Source: CAD feature listing. Evaluate the final solid. Frame: model axes, mm. Round coordinates to 2 decimals unless told otherwise and drop trailing zeros. Write each loop counter-clockwise with the first axis right and the second up, starting at its lowest first coordinate (ties: lowest second). Pieces come first, ordered by that corner, then holes. Notation, with made-up numbers: (59, -7) -> (104, -7) arc R17 cw to (104, 0) -> close; hole circle Ø4 at (0.5, -36.5). An arc over 180 degrees is marked (long way). Put each result on its own line as item: value.
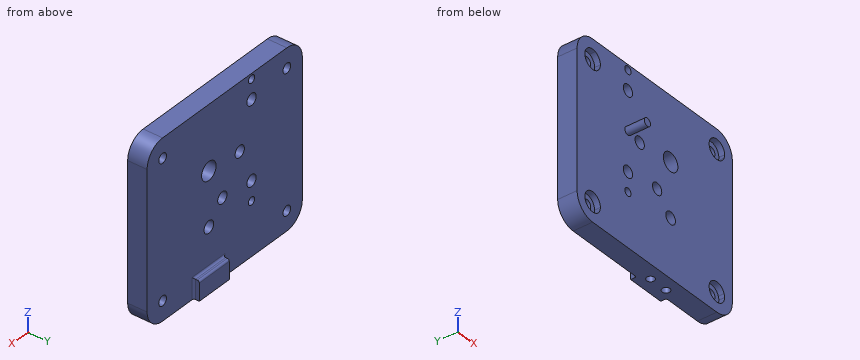
```python
from build123d import *

# Parameters (mm, degrees)
BOSS_EXTRUDE1_DEPTH = 12.7
SKETCH5_R           = 11.9126
SKETCH5_R_2         = 7.9375
SKETCH5_R_3         = 5.9563
CUT_EXTRUDE3_DEPTH  = 231.35713577
CUT_EXTRUDE4_DEPTH  = 231.35713577
CUT_EXTRUDE5_DEPTH  = 7.5057
SKETCH8_R           = 6.35
CUT_EXTRUDE6_DEPTH  = 187.663093698
BOSS_EXTRUDE2_DEPTH = 25.4
SKETCH10_W          = 49.05855317
SKETCH10_H          = 25.4
BOSS_EXTRUDE3_DEPTH = 7.493
FILLET1_R           = 2.54
SKETCH11_R          = 5.08
CUT_EXTRUDE7_DEPTH  = 17.78
SKETCH12_R          = 7.62
CUT_EXTRUDE8_DEPTH  = 188.531502891
SKETCH14_R          = 5.08
BOSS_EXTRUDE4_DEPTH = 50.8
SKETCH16_R          = 7.62
CUT_EXTRUDE10_DEPTH = 193.622803885
SKETCH17_R          = 5.08
CUT_EXTRUDE11_DEPTH = 193.622803885


with BuildPart() as part:
    # Sketch2 → Boss-Extrude1 (new, symmetric)
    with BuildSketch(Plane(origin=(0, 0, 0), x_dir=(1, 0, 0), z_dir=(0, 1, 0))):
        Polygon((114.3, 127), (190.5, 76.2), (190.5, -76.2), (114.3, -127), (-114.3, -127), (-190.5, -76.2), (-190.5, 76.2), (-114.3, 127), align=None)
    extrude(amount=BOSS_EXTRUDE1_DEPTH, both=True)

    # Sketch5 → Cut-Extrude3 (cut, through all)
    # profile 1 of 3: a face of its own
    with BuildSketch(Plane(origin=(0, 12.7, 0), x_dir=(1, 0, 0), z_dir=(0, 1, 0))):
        with Locations(Location((11.947126713, -37.290041101, 0), (0, 0, 270))):
            Circle(SKETCH5_R)
    # profile 2 of 3: a face of its own
    with BuildSketch(Plane(origin=(0, 12.7, 0), x_dir=(1, 0, 0), z_dir=(0, 1, 0))):
        with Locations(Location((11.947126713, 32.712358899, 0), (0, 0, 270))):
            Circle(SKETCH5_R_2)
        with Locations((11.947126713, 32.712358899)):
            Circle(SKETCH5_R_3, mode=Mode.SUBTRACT)
    # profile 3 of 3: a face of its own
    with BuildSketch(Plane(origin=(0, 12.7, 0), x_dir=(1, 0, 0), z_dir=(0, 1, 0))):
        with Locations((11.947126713, 32.712358899)):
            Circle(SKETCH5_R_3)
    extrude(amount=-CUT_EXTRUDE3_DEPTH, mode=Mode.SUBTRACT)

    # Sketch6 → Cut-Extrude4 (cut, through all)
    with BuildSketch(Plane(origin=(0, 12.7, 0), x_dir=(1, 0, 0), z_dir=(0, 1, 0))):
        Polygon((-114.3, -127), (114.3, -127), (190.5, -76.2), (190.5, 76.2), (114.3, 127), (-114.3, 127), (-190.5, 76.2), (-190.5, -76.2), align=None)
        Polygon((-141.354573287, 83.118658899), (-115.954573287, 108.518658899), (87.753426713, 108.518658899), (113.153426713, 83.118658899), (113.153426713, -95.189341101), (87.753426713, -120.589341101), (-115.954573287, -120.589341101), (-141.354573287, -95.189341101), align=None, mode=Mode.SUBTRACT)
    extrude(amount=-CUT_EXTRUDE4_DEPTH, mode=Mode.SUBTRACT)

    # Sketch7 → Cut-Extrude5 (cut)
    with BuildSketch(Plane.XZ.offset(12.7)):
        with BuildLine():
            ThreePointArc((83.29952358, 107.082731992), (78.773170592, 86.20908498), (99.646817604, 90.735437968))
            Line((99.646817604, 90.735437968), (83.29952358, 107.082731992))
        make_face()
        with BuildLine():
            Line((83.29952358, 107.082731992), (99.646817604, 90.735437968))
            ThreePointArc((99.646817604, 90.735437968), (100.250147569, 92.926164607), (100.453426713, 95.189341101))
            ThreePointArc((100.453426713, 95.189341101), (94.989635327, 105.626164607), (83.29952358, 107.082731992))
        make_face()
        with BuildLine():
            ThreePointArc((-103.254573287, 95.189341101), (-105.517749781, 102.425549715), (-111.500670154, 107.082731992))
            Line((-111.500670154, 107.082731992), (-127.847964178, 90.735437968))
            ThreePointArc((-127.847964178, 90.735437968), (-113.691396793, 82.692620245), (-103.254573287, 95.189341101))
        make_face()
        with BuildLine():
            Line((-127.847964178, 90.735437968), (-111.500670154, 107.082731992))
            ThreePointArc((-111.500670154, 107.082731992), (-124.934829408, 104.169597223), (-127.847964178, 90.735437968))
        make_face()
        with BuildLine():
            ThreePointArc((100.453426713, -83.118658899), (100.250147569, -80.855482405), (99.646817604, -78.664755766))
            Line((99.646817604, -78.664755766), (83.29952358, -95.012049789))
            ThreePointArc((83.29952358, -95.012049789), (94.989635327, -93.555482405), (100.453426713, -83.118658899))
        make_face()
        with BuildLine():
            Line((83.29952358, -95.012049789), (99.646817604, -78.664755766))
            ThreePointArc((99.646817604, -78.664755766), (78.773170592, -74.138402777), (83.29952358, -95.012049789))
        make_face()
        with BuildLine():
            ThreePointArc((-127.847964178, -78.664755766), (-124.934829408, -92.09891502), (-111.500670154, -95.012049789))
            Line((-111.500670154, -95.012049789), (-127.847964178, -78.664755766))
        make_face()
        with BuildLine():
            Line((-127.847964178, -78.664755766), (-111.500670154, -95.012049789))
            ThreePointArc((-111.500670154, -95.012049789), (-105.517749781, -90.354867513), (-103.254573287, -83.118658899))
            ThreePointArc((-103.254573287, -83.118658899), (-113.691396793, -70.621938042), (-127.847964178, -78.664755766))
        make_face()
    extrude(amount=-CUT_EXTRUDE5_DEPTH, mode=Mode.SUBTRACT)

    # Sketch8 → Cut-Extrude6 (cut, through all)
    with BuildSketch(Plane.XZ.offset(5.1943)):
        with Locations(Location((-115.954573287, 95.189341101, 0), (0, 0, 270))):
            Circle(SKETCH8_R)
        with Locations(Location((87.753426713, 95.189341101, 0), (0, 0, 270))):
            Circle(SKETCH8_R)
        with Locations(Location((87.753426713, -83.118658899, 0), (0, 0, 270))):
            Circle(SKETCH8_R)
        with Locations(Location((-115.954573287, -83.118658899, 0), (0, 0, 270))):
            Circle(SKETCH8_R)
    extrude(amount=-CUT_EXTRUDE6_DEPTH, mode=Mode.SUBTRACT)

    # Sketch9 → Boss-Extrude2 (add)
    with BuildSketch(Plane(origin=(0, 12.7, 0), x_dir=(1, 0, 0), z_dir=(0, 1, 0))):
        with BuildLine():
            ThreePointArc((113.153426713, 83.118658899), (105.713938955, 101.079171141), (87.753426713, 108.518658899))
            Line((87.753426713, 108.518658899), (113.153426713, 83.118658899))
        make_face()
        with BuildLine():
            ThreePointArc((-115.954573287, 108.518658899), (-133.915085529, 101.079171141), (-141.354573287, 83.118658899))
            Line((-141.354573287, 83.118658899), (-115.954573287, 108.518658899))
        make_face()
        with BuildLine():
            ThreePointArc((-115.954573287, -120.589341101), (-133.915085529, -113.149853344), (-141.354573287, -95.189341101))
            Line((-141.354573287, -95.189341101), (-115.954573287, -120.589341101))
        make_face()
        with BuildLine():
            ThreePointArc((87.753426713, -120.589341101), (105.713938955, -113.149853344), (113.153426713, -95.189341101))
            Line((113.153426713, -95.189341101), (87.753426713, -120.589341101))
        make_face()
    extrude(amount=-BOSS_EXTRUDE2_DEPTH)

    # Sketch10 → Boss-Extrude3 (add)
    with BuildSketch(Plane(origin=(0, 12.7, 0), x_dir=(1, 0, 0), z_dir=(0, 1, 0))):
        with Locations((12.424150128, 95.818658899)):
            Rectangle(SKETCH10_W, SKETCH10_H)
    extrude(amount=BOSS_EXTRUDE3_DEPTH)

    # Fillet1
    fillet1_edges = [part.edges().sort_by_distance(p)[0] for p in [
        (-12.105126457, 12.7, -95.818658899),
        (12.424150128, 12.7, -83.118658899),
        (12.424150128, 20.193, -83.118658899),
        (36.953426713, 12.7, -95.818658899),
    ]]
    fillet(fillet1_edges, radius=FILLET1_R)

    # Sketch11 → Cut-Extrude7 (cut)
    with BuildSketch(Plane(origin=(0, 0, -108.518658899), x_dir=(-1, 0, 0), z_dir=(0, 0, -1))):
        with Locations((0.275849872, 3.7465)):
            Circle(SKETCH11_R)
        with Locations((-25.124150128, 3.7465)):
            Circle(SKETCH11_R)
    extrude(amount=-CUT_EXTRUDE7_DEPTH, mode=Mode.SUBTRACT)

    # Sketch12 → Cut-Extrude8 (cut, through all)
    with BuildSketch(Plane(origin=(0, 12.7, 0), x_dir=(1, 0, 0), z_dir=(0, 1, 0))):
        with Locations(Location((-10.178064282, 8.438679889, 0), (0, 0, 270))):
            Circle(SKETCH12_R)
        with Locations(Location((-38.717702845, -33.586658072, 0), (0, 0, 270))):
            Circle(SKETCH12_R)
    extrude(amount=-CUT_EXTRUDE8_DEPTH, mode=Mode.SUBTRACT)

    # Sketch14 → Boss-Extrude4 (add)
    with BuildSketch(Plane(origin=(0, 12.7, 0), x_dir=(1, 0, 0), z_dir=(0, 1, 0))):
        with Locations(Location((-58.055273287, -37.290041101, 0), (0, 0, 270))):
            Circle(SKETCH14_R)
    extrude(amount=-BOSS_EXTRUDE4_DEPTH)

    # Sketch16 → Cut-Extrude10 (cut, through all)
    with BuildSketch(Plane(origin=(0, 12.7, 0), x_dir=(1, 0, 0), z_dir=(0, 1, 0))):
        with Locations(Location((-58.055273287, 13.509958899, 0), (0, 0, 270))):
            Circle(SKETCH16_R)
        with Locations(Location((-58.055273287, -88.090041101, 0), (0, 0, 270))):
            Circle(SKETCH16_R)
    extrude(amount=-CUT_EXTRUDE10_DEPTH, mode=Mode.SUBTRACT)

    # Sketch17 → Cut-Extrude11 (cut, through all)
    with BuildSketch(Plane(origin=(0, 12.7, 0), x_dir=(1, 0, 0), z_dir=(0, 1, 0))):
        with Locations(Location((-58.055273287, 38.909958899, 0), (0, 0, 270))):
            Circle(SKETCH17_R)
        with Locations(Location((-58.055273287, -113.490041101, 0), (0, 0, 270))):
            Circle(SKETCH17_R)
    extrude(amount=-CUT_EXTRUDE11_DEPTH, mode=Mode.SUBTRACT)


solid = part.part
```
Q1. Cut plane B-B on x = -21. Output: boundary loops of the cut face in (y, z), and give its area (3 significant figures).
Ans:
outline: (-12.7, -108.52) -> (12.7, -108.52) -> (12.7, 120.59) -> (-12.7, 120.59) -> close
area: 5,820 mm^2
Q2. Cut plane C-C on z = 11. Output: boundary loops of the cut face in (x, y).
Ans:
outline: (-141.35, -12.7) -> (113.15, -12.7) -> (113.15, 12.7) -> (-141.35, 12.7) -> close
Q3. Material intervals for line 1 (Z direction, x = -107, y = -12.5); line 2 (Z direction, x = 10, y = -6); line 3 (Y direction, x = -127, z = 108.5), sorted ascending. Write a range as [from, to].
Ans:
line 1: z = [-108.52, -92.12], [-74.11, 86.18], [104.2, 120.59]
line 2: z = [-108.52, -40.41], [-25.02, 25.54], [49.04, 120.59]
line 3: y = [-12.7, 12.7]
Q4. Cut plane A-A on y = -9. Give the number of separate pieces and of enclosed holes in the cut face, and give its area (3 significant figures).
Ans:
separate pieces: 1
enclosed holes: 12
area: 54,200 mm^2
Q5. Pin query (flat end, axial travel): pin 1 (20.5 mm diameter, centred on x = -115.95, z = -83.12, fed in from -Y); pin 2 (6 mm diameter, centred on x = -23.5, z = -55.5, fed in from -Y); pin 3 (0.7 mm diameter, centred on x = 16, y = 17, fed in from +Z). Return the tip coordinate at first contact, or that it passes through.
Ans:
pin 1: stops at y = -5.19
pin 2: stops at y = -12.7
pin 3: stops at z = -83.12
